from build123d import *

# Parameters (mm, degrees)
SKETCH1_W           = 114.3
SKETCH1_H           = 406.4
BOSS_EXTRUDE1_DEPTH = 88.9
SKETCH2_W           = 406.4
SKETCH2_H           = 88.9
BOSS_EXTRUDE2_DEPTH = 114.3
SKETCH3_W           = 76.2
SKETCH3_H           = 101.6
CUT_EXTRUDE1_DEPTH  = 400.05
SKETCH4_W           = 101.6
SKETCH4_H           = 76.2
CUT_EXTRUDE3_DEPTH  = 400.05
SKETCH5_R           = 7.9375
CUT_EXTRUDE4_DEPTH  = 400.05
SKETCH6_R           = 7.9375
CUT_EXTRUDE5_DEPTH  = 400.05


with BuildPart() as part:
    # Sketch1 → Boss-Extrude1 (new body)
    with BuildSketch(Plane.XY):
        Rectangle(SKETCH1_W, SKETCH1_H)
    extrude(amount=BOSS_EXTRUDE1_DEPTH)

    # Sketch2 → Boss-Extrude2 (add)
    with BuildSketch(Plane(origin=(0, 203.2, 0), x_dir=(1, 0, 0), z_dir=(0, 1, 0))):
        with Locations((146.05, -44.45)):
            Rectangle(SKETCH2_W, SKETCH2_H)
    extrude(amount=BOSS_EXTRUDE2_DEPTH)

    # Sketch3 → Cut-Extrude1 (cut)
    with BuildSketch(Plane(origin=(349.25, 0, 0), x_dir=(0, 0, -1), z_dir=(1, 0, 0))):
        with Locations((-44.45, 260.35)):
            Rectangle(SKETCH3_W, SKETCH3_H)
    extrude(amount=-CUT_EXTRUDE1_DEPTH, mode=Mode.SUBTRACT)

    # Sketch4 → Cut-Extrude3 (cut)
    with BuildSketch(Plane.XZ.offset(203.2)):
        with Locations((0, 44.45)):
            Rectangle(SKETCH4_W, SKETCH4_H)
    extrude(amount=-CUT_EXTRUDE3_DEPTH, mode=Mode.SUBTRACT)

    # Sketch5 → Cut-Extrude4 (cut)
    with BuildSketch(Plane.XY.offset(88.9)):
        with Locations((273.05, 260.35)):
            Circle(SKETCH5_R)
        with Locations((95.25, 260.35)):
            Circle(SKETCH5_R)
    extrude(amount=-CUT_EXTRUDE4_DEPTH, mode=Mode.SUBTRACT)

    # Sketch6 → Cut-Extrude5 (cut)
    with BuildSketch(Plane.XY.offset(88.9)):
        with Locations((0, -127)):
            Circle(SKETCH6_R)
        with Locations((0, 50.8)):
            Circle(SKETCH6_R)
    extrude(amount=-CUT_EXTRUDE5_DEPTH, mode=Mode.SUBTRACT)


solid = part.part
Check sheet for the modelled part. Datum: model origin and axes. Units: mm. A direction names the side the tool comes from. Round coordinates to 2 decimals unless told otherwise and drop trailing zeros. Loops run counter-clockwise (first coordinate to the right, second up) from the corner with the lowest first, then second, coordinate; pieces in that order, holes last. Notation, with made-up numbers: M 7.25,-33 L 56.25,-33 A24 ccw 56.25,-15 Z; hole C 67.25,-4.5 d10. An arc over 180 degrees is marked long. One line per question, with ' | ' between items. Start each with the question number.
Item 1: Release check for a two-part mould opening along X. For faces 4 (the face through (267.2, 265.715, 85.769)), 5 (the face through (349.25, 256, 84)), 6 (the face through (152, 260, 6.35)) record: released by +X, released by -X, zero draft, split by the parting line, or undercut.
Item 2: Scan lines: probe 1 along Y at (x, z) = (0, 4.25); probe 2 along X at (y, z) = (260, 2); probe 3 along Y at (x, z) = (300.5, 39). Record each from-to range of solid material in increasing order.
Item 3: Section check D-D (y = -127). Record the boundary of the cut face in (x, z), and give its area (3 significant figures).
Item 4: Section check C-C (x = 273.05). Record the boundary of the cut face in (y, z), and give its area (3 significant figures).
Item 5: Section check B-B (y = 260.35). Record the boundary of the cut face in (x, z).
Item 6: Section check A-A (x = 0). Record the boundary of the cut face in (y, z).
Item 7: Gauge pin test, flat ends, axial feed: pin 1 Ø12 at (x, z) = (294, 64.5) entering from -Y; pin 2 Ø23 at (y, z) = (79.5, 55) entering from +X. Record the tip position at first contact, or that the pin passes through.
Item 8: Set-up check for faces 1 (the face through (-50.8, -6, 44)), 2 (the face through (57.15, -3, 44)), 3 (the face through (152, 209.55, 45)): record each of +Z, -Z, +X, -X, +Y, -Y from which the full face is reachable in a straight line by a thin tool's end or side.
Worked out:
1) face 4: undercut | face 5: released by +X | face 6: zero draft
2) probe 1: -203.2 to -134.94, -119.06 to 42.86, 58.74 to 317.5 | probe 2: -57.15 to 87.32, 103.18 to 265.12, 280.98 to 349.25 | probe 3: 203.2 to 209.55, 311.15 to 317.5
3) outline: M -57.15,0 L -7.94,0 L -7.94,6.35 L -50.8,6.35 L -50.8,82.55 L -7.94,82.55 L -7.94,88.9 L -57.15,88.9 Z; M 7.94,0 L 57.15,0 L 57.15,88.9 L 7.94,88.9 L 7.94,82.55 L 50.8,82.55 L 50.8,6.35 L 7.94,6.35 Z | area: 2,220 mm^2
4) outline: M 203.2,0 L 252.41,0 L 252.41,6.35 L 209.55,6.35 L 209.55,82.55 L 252.41,82.55 L 252.41,88.9 L 203.2,88.9 Z; M 268.29,0 L 317.5,0 L 317.5,88.9 L 268.29,88.9 L 268.29,82.55 L 311.15,82.55 L 311.15,6.35 L 268.29,6.35 Z | area: 2,220 mm^2
5) outline: M -57.15,0 L 87.31,0 L 87.31,6.35 L -50.8,6.35 L -50.8,82.55 L 87.31,82.55 L 87.31,88.9 L -57.15,88.9 Z; M 103.19,0 L 265.11,0 L 265.11,6.35 L 103.19,6.35 Z; M 103.19,82.55 L 265.11,82.55 L 265.11,88.9 L 103.19,88.9 Z; M 280.99,0 L 349.25,0 L 349.25,6.35 L 280.99,6.35 Z; M 280.99,82.55 L 349.25,82.55 L 349.25,88.9 L 280.99,88.9 Z
6) outline: M -203.2,0 L -134.94,0 L -134.94,6.35 L -203.2,6.35 Z; M -203.2,82.55 L -134.94,82.55 L -134.94,88.9 L -203.2,88.9 Z; M -119.06,0 L 42.86,0 L 42.86,6.35 L -119.06,6.35 Z; M -119.06,82.55 L 42.86,82.55 L 42.86,88.9 L -119.06,88.9 Z; M 58.74,0 L 317.5,0 L 317.5,88.9 L 58.74,88.9 L 58.74,82.55 L 196.85,82.55 L 196.85,6.35 L 58.74,6.35 Z; hole M 209.55,6.35 L 311.15,6.35 L 311.15,82.55 L 209.55,82.55 Z
7) pin 1: y = 203.2 | pin 2: x = 57.15
8) face 1: -Y | face 2: +Z, -Z, +X, -Y | face 3: +X
